Work out the finished part from the listing and answer in its coordinate system (mm). Face numbers are marked on the shaded views. A direction names the side the tool comes from. Coordinates: 2 decimals unless noted, no trailing zeros. Loops run counter-clockwise (first coordinate to the right, second up) from the corner with the lowest first, then second, coordinate; pieces in that order, holes last. Notation, with made-up numbers: (-31.75, -34) -> (14.25, -34) arc R32 cw to (14.25, -5) -> close; hole circle Ø11 at (-8, -14). An arc over 180 degrees is marked (long way). Use a Markdown table: item, result.
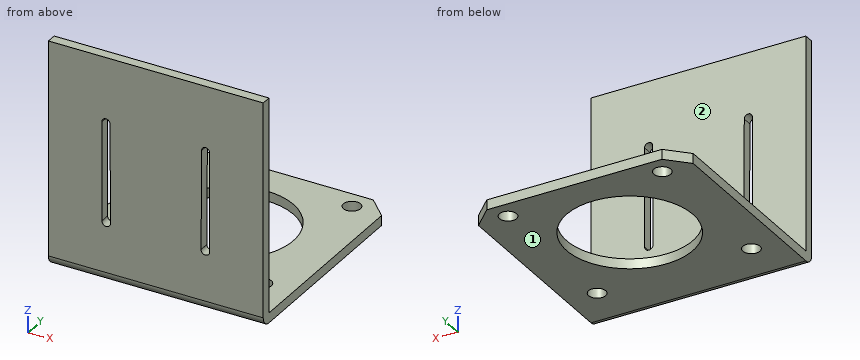
from build123d import *

# Parameters (mm, degrees)
EXTRUDE_1_DEPTH      = 32.5
EXTRUDE_1_DEPTH_BACK = 32.5
FILLET_2_R           = 3
SKETCH_2_R           = 19.1
SKETCH_2_R_2         = 2.6
CUT_EXTRUDE_1_DEPTH  = 13.125
CUT_EXTRUDE_2_DEPTH  = 10


with BuildPart() as part:
    # Sketch 1 → Extrude 1 (new body, two sides)
    with BuildSketch(Plane(origin=(0, 0, 0), x_dir=(0, 0, -1), z_dir=(1, 0, 0))) as extrude_1_sk:
        Polygon((7, 65), (7, -3), (-61, -3), (-61, 0), (4, 0), (4, 65), align=None)
    extrude(amount=EXTRUDE_1_DEPTH)
    extrude(extrude_1_sk.sketch, amount=-EXTRUDE_1_DEPTH_BACK)

    # Fillet 2
    fillet_2_edges = [part.edges().sort_by_distance(p)[0] for p in [
        (0, -3, -7),
    ]]
    fillet(fillet_2_edges, radius=FILLET_2_R)

    # Sketch 2 → Cut-Extrude 1 (cut)
    with BuildSketch(Plane(origin=(0, 0, -7), x_dir=(-1, 0, 0), z_dir=(0, 0, -1))):
        with Locations((0, 36)):
            Circle(SKETCH_2_R)
        with Locations((-23.334523779, 59.334523779)):
            Circle(SKETCH_2_R_2)
        with Locations((23.334523779, 59.334523779)):
            Circle(SKETCH_2_R_2)
        with Locations((23.334523779, 12.665476221)):
            Circle(SKETCH_2_R_2)
        with Locations((-23.334523779, 12.665476221)):
            Circle(SKETCH_2_R_2)
        Polygon((-26.5, 65), (-32.5, 59), (-32.5, 65), align=None)
        Polygon((32.5, 59), (32.5, 65), (26.5, 65), align=None)
    extrude(amount=-CUT_EXTRUDE_1_DEPTH, mode=Mode.SUBTRACT)

    # Sketch 3 → Cut-Extrude 2 (cut)
    with BuildSketch(Plane(origin=(0, 0, 0), x_dir=(1, 0, 0), z_dir=(0, 1, 0))):
        with BuildLine():
            ThreePointArc((-13.695464845, -11.253573908), (-15, -9.949038753), (-16.304535155, -11.253573908))
            Line((-16.304535155, -11.253573908), (-16.304535155, -41.253573908))
            ThreePointArc((-16.304535155, -41.253573908), (-15.08357618, -42.474532883), (-13.862617205, -41.253573908))
            Line((-13.862617205, -41.253573908), (-13.695545839, -11.268110532))
            Line((-13.695545839, -11.268110532), (-13.695464845, -11.253573908))
        make_face()
        with BuildLine():
            Line((16.304535155, -41.253573908), (16.304535155, -11.253573908))
            ThreePointArc((16.304535155, -11.253573908), (15, -9.949038753), (13.695464845, -11.253573908))
            Line((13.695464845, -11.253573908), (13.695545839, -11.268110532))
            Line((13.695545839, -11.268110532), (13.862617205, -41.253573908))
            ThreePointArc((13.862617205, -41.253573908), (15.08357618, -42.474532883), (16.304535155, -41.253573908))
        make_face()
    extrude(amount=-CUT_EXTRUDE_2_DEPTH, mode=Mode.SUBTRACT)


solid = part.part
Q1. Given pin 1 Ø4.5 at (x, y) = (23.33, 12.67) entering from +Z; pin 2 Ø3 at (x, z) = (-5, 11) entering from +Y, each flat-ended and moving along its own axis, determine where each tip first touches the part or whether it passes through.
Solved:
| item | result |
|---|---|
| pin 1 | through |
| pin 2 | y = 0 |
Q2. Section B-B on x = 0 is taken. Determine the outline of the cut face in (y, z), and give its area (3 significant figures).
Solved:
| item | result |
|---|---|
| outline | (-3, -4) arc R3 ccw to (0, -7) -> (16.9, -7) -> (16.9, -4) -> (0, -4) -> (0, 61) -> (-3, 61) -> close; (55.1, -7) -> (65, -7) -> (65, -4) -> (55.1, -4) -> close |
| area | 282 mm² |
Q3. Section C-C on x = -15 is taken. Determine the outline of the cut face in (y, z).
Solved:
| item | result |
|---|---|
| outline | (-3, -4) arc R3 ccw to (0, -7) -> (24.18, -7) -> (24.18, -4) -> (0, -4) -> (0, 9.95) -> (-3, 9.95) -> close; (-3, 42.47) -> (0, 42.47) -> (0, 61) -> (-3, 61) -> close; (47.82, -7) -> (65, -7) -> (65, -4) -> (47.82, -4) -> close |
Q4. Section D-D on z = 49 is taken. Determine the outline of the cut face in (x, y), and give its area (3 significant figures).
Solved:
| item | result |
|---|---|
| outline | (-32.5, -3) -> (32.5, -3) -> (32.5, 0) -> (-32.5, 0) -> close |
| area | 195 mm² |
Q5. For the marked faces 1 and 2, determine the directions among +Z, -Z, +X, -X, +Y, -Y from which every point of the face is accessible in a straight line to the end or side of a thin tool.
Solved:
| item | result |
|---|---|
| face 1 | -Z, +X, -X, +Y, -Y |
| face 2 | +Z, +X, -X, +Y |
Q6. Section A-A on y = 36 is taken. Determine the outline of the cut face in (x, z).
Solved:
| item | result |
|---|---|
| outline | (-32.5, -7) -> (-19.1, -7) -> (-19.1, -4) -> (-32.5, -4) -> close; (19.1, -7) -> (32.5, -7) -> (32.5, -4) -> (19.1, -4) -> close |
Q7. Consider line 1 (Y direction, x = 20, z = 40); line 2 (Z direction, x = -4.5, y = 9). Determine where each line is inside the solid, lowest interval first. Write a range as [from, to].
Solved:
| item | result |
|---|---|
| line 1 | [-3, 0] |
| line 2 | [-7, -4] |
